Read the model definition and answer for the solid it produces. Units are mm, in the model's axes. A direction names the side the tool comes from. Coordinates: 2 decimals unless noted, no trailing zeros. Write each loop counter-clockwise with the first axis right and the second up, starting at its lowest first coordinate (ties: lowest second). Pieces come first, ordered by that corner, then holes.
1) The part is cut by section C-C (z = 1.65). Determine the outline of the cut face in (x, y), then the cut area to 3 significant figures.
2) Find the intervals of material crossed by line 1 (X direction, y = -0.75, z = 0.95); line 2 (Y direction, x = -8, z = 0.9); line 3 (X direction, y = 11, z = 0.85), in increasing order.
3) Each of these flat-tipped pins is pushed along its axis until it touches: pin 1 Ø1.6 at (x, y) = (8, 0) entering from +Z; pin 2 Ø3 at (x, y) = (-8, 0) entering from +Z; pin 3 Ø1 at (x, z) = (-5.5, 2) entering from +Y. Where does it stop, or does it pass through?
4) Determine the mould class of faces 1 (the face through (8, 3.5, 1)), 2 (the face through (-7.2, 0.6, 1)), 3 (the face through (-3.5, 9, 1)) for opening direction X: +X half, -X half, draft (parallel to the pull), parting line (faces both ways), or undercut.
5) Which of the six approach directions +Z, -Z, +X, -X, +Y, -Y give full straight-line access (tool end or side, diameter ignored) to faces 4 (the face through (3.5, 9, 1)), 5 (the face through (-8, 3.5, 1)), 6 (the face through (0, -3.5, 1))?
6) The part is cut by section D-D (y = 10.5). Determine the outline of the cut face in (x, z), then the cut area to 3 significant figures.
7) The part is cut by section A-A (x = 8). Determine the outline of the cut face in (y, z).
8) The part is cut by section B-B (y = 0). Determine the outline of the cut face in (x, z).
from build123d import *

# Parameters (mm, degrees)
F1_DEPTH = 2
F2_D     = 2


with BuildPart() as f1:
    # F0 (on Top) → F1 (new body)
    with BuildSketch(Plane.XY):
        Polygon((-9.9, -3.5), (9.9, -3.5), (9.9, 3.5), (5.5, 3.5), (3.5, 3.5), (-3.5, 3.5), (-5.5, 3.5), (-9.9, 3.5), align=None)
        Polygon((-3.5, 3.5), (3.5, 3.5), (3.5, 5.5), (3.5, 12.5), (-3.5, 12.5), (-3.5, 5.5), align=None)
        with BuildLine():
            ThreePointArc((-3.5, 5.5), (-4.085786, 4.085786), (-5.5, 3.5))
            Line((-5.5, 3.5), (-3.5, 3.5))
            Line((-3.5, 3.5), (-3.5, 5.5))
        make_face()
        with BuildLine():
            Line((3.5, 3.5), (5.5, 3.5))
            ThreePointArc((5.5, 3.5), (4.085786, 4.085786), (3.5, 5.5))
            Line((3.5, 5.5), (3.5, 3.5))
        make_face()
    extrude(amount=F1_DEPTH)

    # F2 (through all)
    with Locations(Plane(origin=(0, 0, 0), x_dir=(1, 0, 0), z_dir=(0, 0, -1))):
        with Locations((-8, 0), (8, 0)):
            Hole(F2_D / 2)


solid = f1.part
Reported:
1. outline: (-9.9, -3.5) - (9.9, -3.5) - (9.9, 3.5) - (5.5, 3.5) arc R2 cw to (3.5, 5.5) - (3.5, 12.5) - (-3.5, 12.5) - (-3.5, 5.5) arc R2 cw to (-5.5, 3.5) - (-9.9, 3.5) - close; hole circle Ø2 at (-8, 0); hole circle Ø2 at (8, 0)
1. area: 197 mm2
2. line 1: x = -9.9 to -8.66, -7.34 to 7.34, 8.66 to 9.9
2. line 2: y = -3.5 to -1, 1 to 3.5
2. line 3: x = -3.5 to 3.5
3. pin 1: passes through
3. pin 2: stops at z = 2
3. pin 3: stops at y = 3.56
4. face 1: draft
4. face 2: undercut
4. face 3: -X half
5. face 4: +Z, -Z, +X, +Y
5. face 5: +Z, -Z, -X, +Y
5. face 6: +Z, -Z, +X, -X, -Y
6. outline: (-3.5, 0) - (3.5, 0) - (3.5, 2) - (-3.5, 2) - close
6. area: 14.0 mm2
7. outline: (-3.5, 0) - (-1, 0) - (-1, 2) - (-3.5, 2) - close; (1, 0) - (3.5, 0) - (3.5, 2) - (1, 2) - close
8. outline: (-9.9, 0) - (-9, 0) - (-9, 2) - (-9.9, 2) - close; (-7, 0) - (7, 0) - (7, 2) - (-7, 2) - close; (9, 0) - (9.9, 0) - (9.9, 2) - (9, 2) - close
